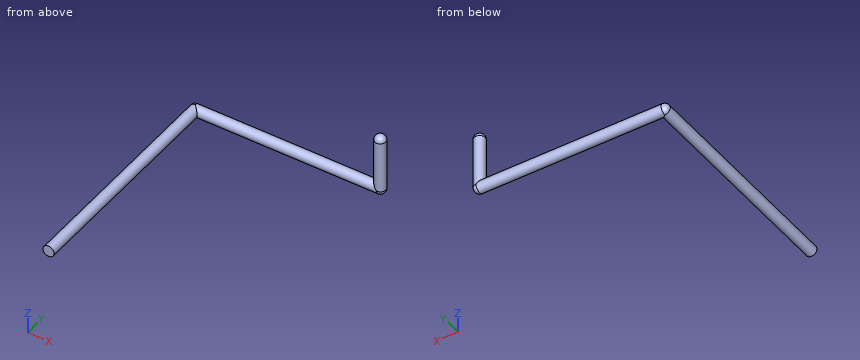
from build123d import *

# Parameters (mm, degrees)
SKETCH_1_R      = 0.75
EXTRUDE_1_DEPTH = 30
SKETCH_3_R      = 0.75
EXTRUDE_2_DEPTH = 25
SKETCH_5_R      = 0.75
EXTRUDE_3_DEPTH = 7


with BuildPart() as part:
    # 草图1 → 凸台-拉伸1 (new body)
    with BuildSketch(Plane(origin=(0, 0, 0), x_dir=(1, 0, 0), z_dir=(0, 1, 0))):
        with Locations(Location((0, 0, 0), (0, 0, 270))):
            Circle(SKETCH_1_R)
    extrude(amount=EXTRUDE_1_DEPTH)

    # 草图2 → 旋转1 (revolve)
    with BuildSketch(Plane(origin=(0, 0, 0), x_dir=(0, 0, -1), z_dir=(1, 0, 0))):
        with BuildLine():
            Line((0, 30.75), (0, 29.25))
            ThreePointArc((0, 29.25), (0.75, 30), (0, 30.75))
        make_face()
    revolve(axis=Axis((0, 30.75, 0), (0, -1, 0)))

    # 草图3 → 凸台-拉伸2 (add)
    with BuildSketch(Plane(origin=(0, 0, 0), x_dir=(0, 0, -1), z_dir=(1, 0, 0))):
        with Locations((0, 30)):
            Circle(SKETCH_3_R)
    extrude(amount=EXTRUDE_2_DEPTH)

    # 草图4 → 旋转2 (revolve)
    with BuildSketch(Plane.XY):
        with BuildLine():
            Line((24.25, 30), (25.75, 30))
            ThreePointArc((25.75, 30), (25, 30.75), (24.25, 30))
        make_face()
    revolve(axis=Axis((24.25, 30, 0), (1, 0, 0)))

    # 草图5 → 凸台-拉伸3 (add)
    with BuildSketch(Plane.XY):
        with Locations((25, 30)):
            Circle(SKETCH_5_R)
    extrude(amount=EXTRUDE_3_DEPTH)

    # 草图6 → 旋转3 (revolve)
    with BuildSketch(Plane.XY.offset(7)):
        with BuildLine():
            Line((25, 30.75), (25, 29.25))
            ThreePointArc((25, 29.25), (25.75, 30), (25, 30.75))
        make_face()
    revolve(axis=Axis((25, 30.75, 7), (0, -1, 0)))


solid = part.part
Read the model definition and answer for the solid it produces. Units are mm, in the model's axes. Coordinates: 2 decimals unless noted, no trailing zeros. Order: outer loops, then holes, each group sorted by start corner. A loop starts at its lowest first (then second) coordinate and runs counter-clockwise, first axis right, second up. Notation, with made-up numbers: M -23.5,-22.75 L 11.5,-22.75 A6 ccw 11.5,-18.75 Z; hole C 49,4 d2. An arc over 180 degrees is marked long. Put each result on its own line as item: value. Start each with the question number.
Item 1: Consider probe 1 along Z at (x, y) = (17.5, 30); probe 2 along Y at (x, z) = (9.5, 0). Determine where each line is inside the solid, lowest interval first. Write a range as [from, to].
Item 2: Given pin 1 Ø1.5 at (x, z) = (22.5, 3.5) entering from -Y, flat-ended and moving along its own axis, determine where the tip first touches the part or whether it passes through.
Item 3: Section B-B, the plane z = 3 is taken. Determine the outline of the cut face in (x, y).
Item 4: Section A-A, the plane y = 24.5 is taken. Determine the outline of the cut face in (x, z), plus the area to 3 significant figures.
Computed:
1. probe 1: z = [-0.75, 0.75]
1. probe 2: y = [29.25, 30.75]
2. pin 1: passes through
3. outline: C 25,30 d1.5
4. outline: C 0,0 d1.5
4. area: 1.77 mm2
